```python
from build123d import *

# Parameters (mm, degrees)
SKETCH1_R           = 14.2
BOSS_EXTRUDE1_DEPTH = 59
SKETCH2_R           = 2
BOSS_EXTRUDE2_DEPTH = 17.8
SKETCH3_R           = 1.5
CUT_EXTRUDE1_DEPTH  = 4.3942
SKETCH5_W           = 1.529717974
SKETCH5_H           = 4.18122913
CUT_EXTRUDE2_DEPTH  = 13.716


with BuildPart() as part:
    # Sketch1 → Boss-Extrude1 (new body)
    with BuildSketch(Plane.XY):
        Circle(SKETCH1_R)
    extrude(amount=BOSS_EXTRUDE1_DEPTH)

    # Sketch2 → Boss-Extrude2 (add)
    with BuildSketch(Plane.XY.offset(59)):
        Circle(SKETCH2_R)
    extrude(amount=BOSS_EXTRUDE2_DEPTH)

    # Sketch3 → Cut-Extrude1 (cut)
    with BuildSketch(Plane.XY.offset(59)):
        with Locations((-8.5, 0)):
            Circle(SKETCH3_R)
        with Locations((8.5, 0)):
            Circle(SKETCH3_R)
    extrude(amount=-CUT_EXTRUDE1_DEPTH, mode=Mode.SUBTRACT)

    # Sketch5 → Cut-Extrude2 (cut)
    with BuildSketch(Plane.XY.offset(63.5)):
        with Locations((-1.886652168, -0.050990599)):
            Rectangle(SKETCH5_W, SKETCH5_H)
    extrude(amount=CUT_EXTRUDE2_DEPTH, mode=Mode.SUBTRACT)


solid = part.part
```
Work out the finished part from the listing and answer in its coordinate system (mm). A direction names the side the tool comes from. Round coordinates to 2 decimals unless told otherwise and drop trailing zeros. Write each loop counter-clockwise with the first axis right and the second up, starting at its lowest first coordinate (ties: lowest second). Pieces come first, ordered by that corner, then holes. Notation, with made-up numbers: (-4, 20) - (1, 20) arc R23 ccw to (1, 52) - close; hole circle Ø2 at (36.5, 33.5). An arc over 180 degrees is marked (long way). Return JSON: item names as keys, results as strings. Group by question number.
Q1. Each of these flat-tipped pins is pushed along its axis until it touches: pin 1 Ø1.5 at (x, y) = (9, 0.5) entering from +Z; pin 2 Ø5 at (x, z) = (-3.5, 33.5) entering from -Y; pin 3 Ø1.7 at (y, z) = (-0.5, 68) entering from -X. Where does it stop, or does it pass through?
Q2. The mould has two halves that part along Y. Classify faces 1 (the cylindrical face through (-1.85, 14.08, 29.09)), 2 (the flat face through (-9, 0, 54.606)), 3 (the flat face through (3, 0, 59)), 4 (the cylindrical face through (7.3, -0.9, 56.8)): released by +Y, released by -Y, zero draft, split by the parting line, or undercut.
Q3. The part is cut by section A-A on y = 0. Write down the section's boundary in (x, z), then the cut area to 3 significant figures.
Q4. The part is cut by section D-D on x = 8.5. Write down the section's boundary in (y, z).
Q5. The part is cut by section B-B on x = 0. Write down the section's boundary in (y, z), then the cut area to 3 significant figures.
Q6. The part is cut by section C-C on z = 35. Write down the section's boundary in (x, y), then the cut area to 3 significant figures.
Q7. For faces 5 (the flat face through (0, 0, 0)), 6 (the flat face through (8, 0, 54.606)), 7 (the flat face through (-1.122, 0, 70)), determine the directions among +Z, -Z, +X, -X, +Y, -Y from which every point of the face is accessible in a straight line to the end or side of a thin tool.
Q8. Find the intervals of material crossed by L1, parallel to Z at x = -2.75, y = 6; L2, parallel to Y at x = -8.5, z = 57.55; L3, parallel to Y at x = -11, z = 19.5, in increasing order.
Solved:
{
 "1": {"pin 1": "z = 54.61", "pin 2": "y = -14.16", "pin 3": "x = -1.12"},
 "2": {"face 1": "split by the parting line", "face 2": "undercut", "face 3": "zero draft", "face 4": "undercut"},
 "3": {"outline": "(-14.2, 0) - (14.2, 0) - (14.2, 59) - (10, 59) - (10, 54.61) - (7, 54.61) - (7, 59) - (2, 59) - (2, 76.8) - (-1.12, 76.8) - (-1.12, 63.5) - (-2, 63.5) - (-2, 59) - (-7, 59) - (-7, 54.61) - (-10, 54.61) - (-10, 59) - (-14.2, 59) - close", "area": "1,710 mm²"},
 "4": {"outline": "(-11.37, 0) - (11.37, 0) - (11.37, 59) - (1.5, 59) - (1.5, 54.61) - (-1.5, 54.61) - (-1.5, 59) - (-11.37, 59) - close"},
 "5": {"outline": "(-14.2, 0) - (14.2, 0) - (14.2, 59) - (2, 59) - (2, 76.8) - (-2, 76.8) - (-2, 59) - (-14.2, 59) - close", "area": "1,750 mm²"},
 "6": {"outline": "circle Ø28.4 at (0, 0)", "area": "633 mm²"},
 "7": {"face 5": "-Z, +X, -X, +Y, -Y", "face 6": "+Z", "face 7": "+Z, -X, +Y, -Y"},
 "8": {"L1": "0 to 59", "L2": "-11.37 to -1.5, 1.5 to 11.37", "L3": "-8.98 to 8.98"}
}
